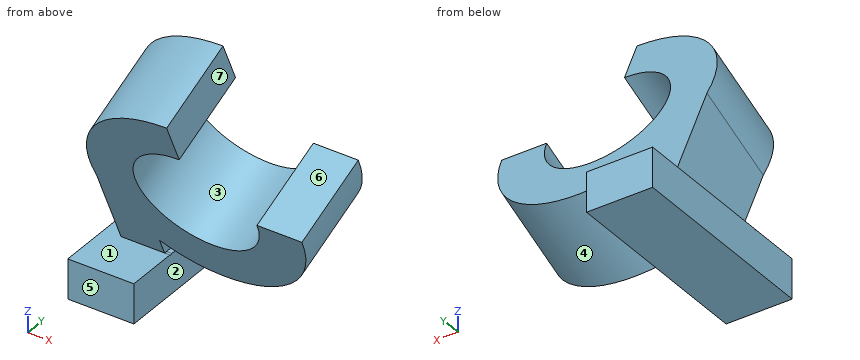
from build123d import *

# Parameters (mm, degrees)
F2_R      = 40
F2_R_2    = 23
F4_DEPTH  = 34
F8_DEPTH  = 25
F11_DEPTH = 34
F12_DEPTH = 25
F13_DEPTH = 180.6
F15_DEPTH = 6.54


with BuildPart() as f4:
    # F2 (on line) → F4 (new body)
    with BuildSketch(Plane(origin=(0, 0, 0), x_dir=(-1, 0, 0), z_dir=(0, 0.9135454576, 0.4067366431))):
        Circle(F2_R)
        Circle(F2_R_2, mode=Mode.SUBTRACT)
    extrude(amount=-F4_DEPTH)



with BuildPart() as f8:
    # F7 (on offset) → F8 (new body)
    with BuildSketch(Plane.YZ.offset(-46)):
        Polygon((-14.7910798368, -50.3708641703), (-14.9561992038, -50), (-34.7910798368, -50), (-34.7910798368, -65), (-14.7910798368, -65), align=None)
        Polygon((42.1320945024, -50), (22.2614342654, -50), (28.9398645451, -65), (42.1320945024, -65), align=None)
        Polygon((22.2614342654, -50), (0, -50), (0, -65), (28.9398645451, -65), align=None)
        Polygon((-8.2777689242, -65), (-14.7910798368, -50.3708641703), (-14.7910798368, -65), align=None)
        Polygon((0, -65), (0, -50), (-13.9581052722, -50), (-14.7910798368, -50.3708641703), (-8.2777689242, -65), align=None)
    extrude(amount=F8_DEPTH)


with BuildPart() as f4_1:
    add(f4.part)

    add(f8.part)  # F11 merges F8
    # F10 (on face) → F11 (join, through all)
    with BuildSketch(Plane(origin=(0, 0, 0), x_dir=(-1, 0, 0), z_dir=(0, 0.9135454576, 0.4067366431))):
        with BuildLine():
            ThreePointArc((39.4592955709, -6.5546924453), (33.8604048962, -21.2949050306), (23, -32.7261363439))
            Line((23, -32.7261363439), (23, -83.8858187199))
            Line((23, -83.8858187199), (39.4592955709, -83.8858187199))
            Line((39.4592955709, -83.8858187199), (39.4592955709, -6.5546924453))
        make_face()
    extrude(amount=-F11_DEPTH)

    # F12 (cut): a face of the model
    f12_faces = [f4_1.faces().sort_by_distance(p)[0] for p in [
        (-39.4592955709, 12.3389864526, -74.7036267653),
    ]]
    extrude(f12_faces, amount=-F12_DEPTH, mode=Mode.SUBTRACT)

    # F9 (on line) → F13 (cut)
    with BuildSketch(Plane(origin=(0, 0, 0), x_dir=(-1, 0, 0), z_dir=(0, 0.9135454576, 0.4067366431))):
        with BuildLine():
            Line((0, 23), (0, 40))
            ThreePointArc((0, 40), (-28.2842712475, 28.2842712475), (-40, 0))
            Line((-40, 0), (-23, 0))
            ThreePointArc((-23, 0), (-16.2634559673, 16.2634559673), (0, 23))
        make_face()
    extrude(amount=-F13_DEPTH, mode=Mode.SUBTRACT)

    # F14 (on face) → F15 (join)
    with BuildSketch(Plane(origin=(-39.4592955709, 0, 0), x_dir=(0, -1, 0), z_dir=(-1, 0, 0))):
        Polygon((14.7910798368, -50.3708641703), (14.9561992038, -50), (13.9581052722, -50), align=None)
    extrude(amount=F15_DEPTH)


solid = f4_1.part
Input: part model. Units: mm. Frame: model coordinates. Face numbers are marked on the shaded views. A direction names the side the tool comes from. Give positions to 0.01 mm unless a question says otherwise; leave off trailing zeros. Loops run counter-clockwise (first coordinate to the right, second up) from the corner with the lowest first, then second, coordinate; pieces in that order, holes last. Notation, with made-up numbers: (-32.5, -2) - (-18.5, -2) arc R32 cw to (-18.5, 33) - close; hole circle Ø11 at (33.5, -28). An arc over 180 degrees is marked (long way). Use CSV: the item, a comma, the result in double quotes. Start each with the question number.
Item 1: Section C-C on y = 26. Return loops of the section in (x, z), then the cut area to 3 significant figures.
Item 2: Reachability of the marked faces 5, 6 and 7 from +Z, -Z, +X, -X, +Y, -Y: full face, straight path, thin tool, end or side. Return the list, or none.
Item 3: Contact query for flat-ended pins moving along their axis: P1, Ø10, axis at x = 6.5, z = 9, coming from the +Y side; P2, Ø4.5, axis at x = -29.5, z = -59.5, coming from the -Y side; P3, Ø13, axis at y = -14.5, z = -20.5, coming from the -X side; P4, Ø14.5, axis at y = -23, z = 25, coming from the +X side. Output: stop coordinate, or through.
Item 4: Section D-D on y = -23. State how many separate pieces and enclosed holes the cut face has, then the cut area to 3 significant figures.
Item 5: Mould query, pull axis X, two halves, no side actions, for the marked faces 1, 2, 3 and 4. Classes: pulls with the +X half, pulls with the -X half, needs draft (parallel to the pull), parting line crosses it, or undercut.
Item 6: Section A-A on x = -17.5. Return loops of the section in (y, z).
Item 7: Section B-B on x = -33. Return loops of the section in (y, z), then the cut area to 3 significant figures.
Item 8: Line query: line 1 (Z direction, x = -34, y = 26.5); line 2 (Z direction, x = -32.5, y = -34.5); line 3 (X direction, y = 1, z = -52). Output: solid intervals per line, ascending.
Ans:
1,outline,"(-46, -65) - (-21, -65) - (-21, -50) - (-46, -50) - close"
1,area,"375 mm2"
2,face 5,"-Z, +X, -X, -Y"
2,face 6,"+Z, +X, -Y"
2,face 7,"+Z, +X, +Y, -Y"
3,P1,"passes through"
3,P2,"stops at y = -34.79"
3,P3,"stops at x = -39.5"
3,P4,"stops at x = 0"
4,separate pieces,"3"
4,enclosed holes,"0"
4,area,"2,130 mm2"
5,face 1,"needs draft"
5,face 2,"pulls with the +X half"
5,face 3,"undercut"
5,face 4,"undercut"
6,outline,"(-45.69, 19.03) - (-37.13, -0.19) - (-6.07, 13.63) - (-14.63, 32.86) - close; (-24.99, -27.46) - (-16.43, -46.69) - (14.63, -32.86) - (6.07, -13.63) - close"
7,outline,"(-40.25, 6.82) - (-14.96, -50) - (-34.79, -50) - (-34.79, -65) - (42.13, -65) - (42.13, -50) - (22.26, -50) - (-9.19, 20.65) - close"
7,area,"3,530 mm2"
8,line 1,"z = -65 to -50"
8,line 2,"z = -65 to -50, -6.1 to 10.16"
8,line 3,"x = -46 to -21"
